Check sheet for the drawn part. Datum: minimum x, y, z corner. Units: mm. A direction names the side the tool comes from. Coordinates: 2 decimals unless noted, no trailing zeros. Order: outer loops, then holes, each group sorted by start corner. A loop starts at its lowest first (then second) coordinate and runs counter-clockwise, first axis right, second up. Notation, with made-up numbers: M -34.75,-16 L 5.25,-16 A29 cw 5.25,6 Z; hole C 44.5,-7.5 d3. An arc over 180 degrees is marked long. Answer in a Markdown table with one row per item. Add a question column.
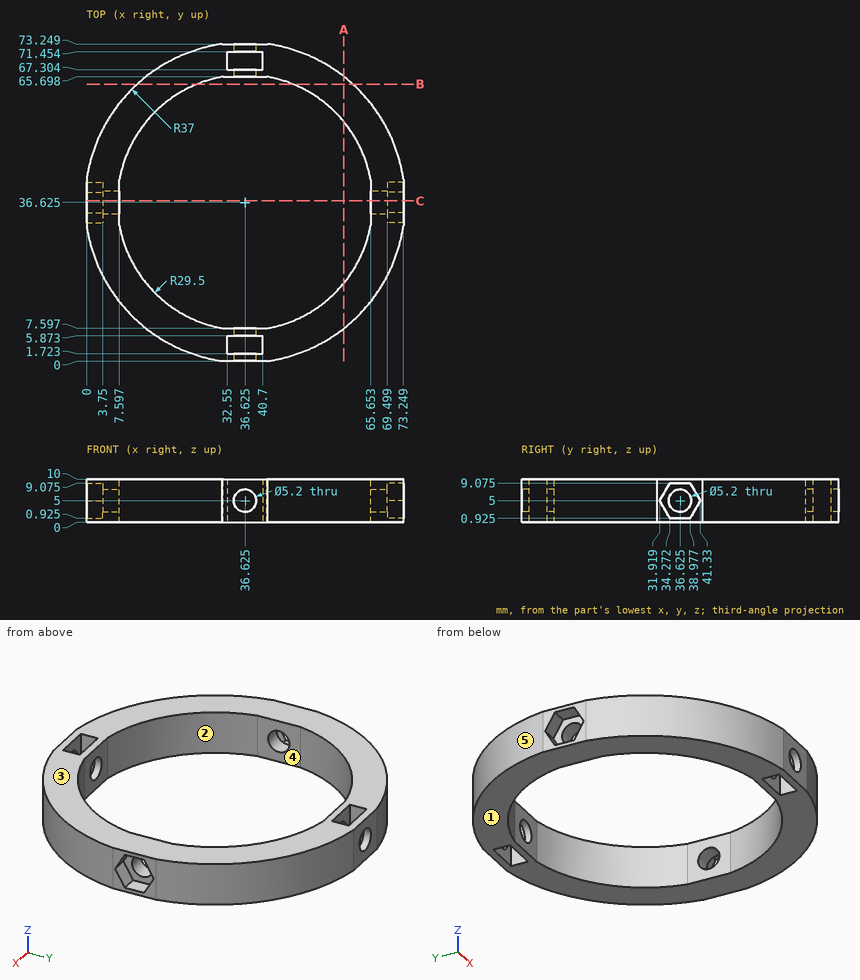
1. Set-up check for the marked faces 1 and 2: record each of +Z, -Z, +X, -X, +Y, -Y from which the full face is reachable in a straight line by a thin tool's end or side.
2. Section check A-A on x = 59.5. Enter the section's corners in (y, z), then the cut area to 3 significant figures.
3. Go/stop test with flat-tipped pins: pin 1 Ø3.5 at (y, z) = (69.5, 7.5) entering from +X; pin 2 Ø5 at (y, z) = (21.5, 2.5) entering from -X (1 decimal); pin 3 Ø4 at (y, z) = (36, 7) entering from +X. Record where each tip stops, or that it passes through.
4. Section check C-C on y = 37. State how many separate pieces and enclosed holes the cut face has.
5. Section check B-B on y = 64. Enter the section's corners in (x, z).
6. Scan lines: line 1 (Y direction, x = 3, z = 6.5) (1 decimal); line 2 (X direction, y = 7, z = 5.25) (1 decimal); line 3 (X direction, y = 10.5, z = 2.5) (1 decimal). Record each from-to range of solid material in increasing order.
7. Release check for a two-part mould opening along Y. For the marked faces 3, 4 and 5 record: released by +Y, released by -Y, zero draft, split by the parting line, or undercut.
Result sheet:
| question | item | result |
|---|---|---|
| 1 | face 1 | -Z, +X, -X, +Y, -Y |
| 1 | face 2 | +Z, -Z |
| 2 | outline | M 7.54,0 L 18,0 L 18,10 L 7.54,10 Z; M 55.25,0 L 65.71,0 L 65.71,10 L 55.25,10 Z |
| 2 | area | 209 mm^2 |
| 3 | pin 1 | x = 56.63 |
| 3 | pin 2 | x = 1.8 |
| 3 | pin 3 | x = 69.5 |
| 4 | separate pieces | 4 |
| 4 | enclosed holes | 0 |
| 5 | outline | M 11.73,0 L 25.63,0 L 25.63,10 L 11.73,10 Z; M 47.62,0 L 61.52,0 L 61.52,10 L 47.62,10 Z |
| 6 | line 1 | 21.2 to 32.8, 40.5 to 52.1 |
| 6 | line 2 | 14.5 to 34, 39.2 to 58.8 |
| 6 | line 3 | 10.4 to 22.9, 50.3 to 62.8 |
| 7 | face 3 | zero draft |
| 7 | face 4 | undercut |
| 7 | face 5 | released by +Y |
